Here's how the part is built. I have some questions about the finished solid (model axes, mm). Face numbers are marked on the shaded views. A direction names the side the tool comes from. Give positions to 0.01 mm unless a question says otherwise; leave off trailing zeros. Write each loop counter-clockwise with the first axis right and the second up, starting at its lowest first coordinate (ties: lowest second). Pieces come first, ordered by that corner, then holes. Notation, with made-up numbers: (76, 53.5) - (94, 53.5) arc R24 ccw to (94, 83.5) - close; hole circle Ø11 at (-18.5, 45). An arc over 180 degrees is marked (long way). One line per item, written item: value. Start each with the question number.
1) Imagine slicing it at A-A on x = 62.5. Write out the boundary of the cut face in (y, z).
2) Imagine slicing it at C-C on y = -21. Write out the boundary of the cut face in (x, z), plus the area to 3 significant figures.
3) On a 3-axis mill with a long thin cutter (end or side, diameter ignored), from which of +Z, -Z, +X, -X, +Y, -Y can I reach the whole of each face in a straight line? I mean the marked faces 4 and 5. Say none if no direction works.
4) Please list where these lines run through material, in increasing order: L1, parallel to Y at x = -0.95, z = 0; L2, parallel to Y at x = 6, z = 0; L3, parallel to Z at x = 6, y = -21. Write a range as [from, to].
5) Imagine slicing it at B-B on y = 42. Write out the boundary of the cut face in (x, z).
6) We'd pull the mould along Y, two halves only. Please class the marked faces 1, 2 and 3: +Y half, -Y half, draft (parallel to the pull), parting line (faces both ways), or undercut.
7) Imagine slicing it at D-D on z = -27. Write out the boundary of the cut face in (x, y), plus the area to 3 significant figures.
8) I'm going to push flat-ended pins straight in: P1, Ø1.4, axis at x = 64, y = 7, coming from the -Z side; P2, Ø13.5, axis at y = -3.5, z = -0.5, coming from the -X side; P3, Ø1.3, axis at x = 66.5, z = -1, coming from the +Y side; P4, Ø4.5, axis at y = 29, z = 0, coming from the -X side. Where does each tip first touch, or does it pass through?
from build123d import *

# Parameters (mm, degrees)
ESQUISSE3_R             = 3
ENL_V_MAT_EXTRU_1_DEPTH = 102.901913623
ESQUISSE7_R             = 3
ENL_V_MAT_EXTRU_2_DEPTH = 102.901913623
TROU_TARAUD_M63_D       = 5
TROU_TARAUD_M63_DEPTH   = 15
TROU_TARAUD_M63_TIP     = 1.502151548
D_GAGEMENT_M37_REACH    = 105.064
D_GAGEMENT_M37_BORE_R   = 1.7
ESQUISSE6_W             = 10.447703872
ESQUISSE6_H             = 4.5
ENL_V_MAT_EXTRU_3_DEPTH = 2
D_GAGEMENT_M51_D        = 5.5
D_GAGEMENT_M51_DEPTH    = 12
D_GAGEMENT_M51_TIP      = 1.652366702


with BuildPart() as part:
    # Esquisse1 → Révolution2 (revolve)
    with BuildSketch(Plane.XY, mode=Mode.PRIVATE) as r_volution2_sk:
        with BuildLine():
            Line((0, 0), (74.5, 0))
            Line((74.5, 0), (74.5, -6))
            Line((74.5, -6), (69.5, -6))
            Line((69.5, -6), (69.5, -7))
            Line((69.5, -7), (68, -8.5))
            Line((68, -8.5), (60.5, -8.5))
            Line((60.5, -8.5), (60.5, -7.5))
            Line((60.5, -7.5), (59.5, -7.5))
            Line((59.5, -7.5), (59.5, -10))
            Line((59.5, -10), (13, -10))
            ThreePointArc((13, -10), (12.646446609, -10.146446609), (12.5, -10.5))
            Line((12.5, -10.5), (12.5, -13.5))
            Line((12.5, -13.5), (8.5, -17))
            Line((8.5, -17), (8.5, -48))
            Line((8.5, -48), (-1.5, -48))
            Line((-1.5, -48), (-1.5, -35))
            Line((-1.5, -35), (0, -35))
            Line((0, -35), (0, 0))
        make_face()
    revolve(r_volution2_sk.sketch.rotate(Axis((-50.843487897, 0, 0), (1, 0, 0)), 270), axis=Axis((-50.843487897, 0, 0), (1, 0, 0)))

    # Esquisse2 → Dégagement M32 (revolve, cut)
    with BuildSketch(Plane(origin=(74.5, 0, 0), x_dir=(0, 0, -1), z_dir=(0, 1, 0))):
        Polygon((0, 0), (0, 14.981495458), (1.7, 14), (1.7, 0), align=None)
    revolve(axis=Axis((80.85, 0, 0), (-1, 0, 0)), mode=Mode.SUBTRACT)

    # Esquisse3 → Enlèv. mat.-Extru.1 (cut, through all)
    with BuildSketch(Plane.ZY.offset(1.5)):
        with Locations((-40, 0)):
            Circle(ESQUISSE3_R)
        with Locations((40, 0)):
            Circle(ESQUISSE3_R)
    extrude(amount=-ENL_V_MAT_EXTRU_1_DEPTH, mode=Mode.SUBTRACT)

    # Esquisse7 → Enlèv. mat.-Extru.2 (cut, through all)
    with BuildSketch(Plane.ZY.offset(1.5)):
        with Locations((0, -44)):
            Circle(ESQUISSE7_R)
    extrude(amount=-ENL_V_MAT_EXTRU_2_DEPTH, mode=Mode.SUBTRACT)

    # Trou taraudé M63
    with Locations(Plane(origin=(-1.5, 42, 0), x_dir=(0, 0, -1), z_dir=(-1, 0, 0))):
        with Locations((0, 0), (36.373066959, 63), (-36.373066959, 63)):
            Hole(TROU_TARAUD_M63_D / 2, depth=TROU_TARAUD_M63_DEPTH)
            with Locations((0, 0, -(TROU_TARAUD_M63_DEPTH + TROU_TARAUD_M63_TIP / 2))):  # 118° drill point
                Cone(0, TROU_TARAUD_M63_D / 2, TROU_TARAUD_M63_TIP, mode=Mode.SUBTRACT)

    # Dégagement M37 bore (on position points) → Dégagement M37 (cut, up to next)
    with BuildSketch(Plane(origin=(72, 6, 0), x_dir=(0, 0, 1), z_dir=(0, 1, 0)), mode=Mode.PRIVATE) as d_gagement_m37_sk1:
        Circle(D_GAGEMENT_M37_BORE_R)
    d_gagement_m37_tool1 = extrude(d_gagement_m37_sk1.sketch, amount=-D_GAGEMENT_M37_REACH, mode=Mode.PRIVATE) & part.part
    add(d_gagement_m37_tool1.solids().sort_by_distance((72, 6, 0))[0], mode=Mode.SUBTRACT)

    # Esquisse6 → Enlèv. mat.-Extru.3 (cut)
    with BuildSketch(Plane(origin=(0, 8.5, 0), x_dir=(-1, 0, 0), z_dir=(0, 1, 0))):
        with Locations((-65.723851936, 0)):
            Rectangle(ESQUISSE6_W, ESQUISSE6_H)
    extrude(amount=-ENL_V_MAT_EXTRU_3_DEPTH, mode=Mode.SUBTRACT)

    # Dégagement M51
    with Locations(Plane(origin=(8.5, 29, 0), x_dir=(0, 0, 1), z_dir=(1, 0, 0))):
        with Locations((0, 0)):
            Hole(D_GAGEMENT_M51_D / 2, depth=D_GAGEMENT_M51_DEPTH)
            with Locations((0, 0, -(D_GAGEMENT_M51_DEPTH + D_GAGEMENT_M51_TIP / 2))):  # 118° drill point
                Cone(0, D_GAGEMENT_M51_D / 2, D_GAGEMENT_M51_TIP, mode=Mode.SUBTRACT)


solid = part.part
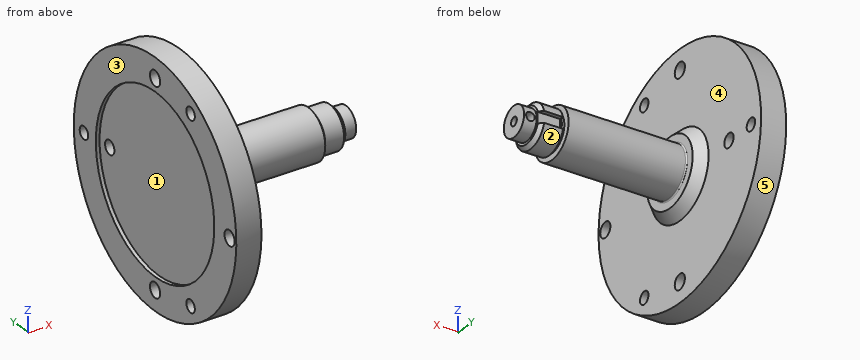
Numbers:
1. outline: (6.5, -2.25) - (6.5, 2.25) - (8.2, 2.25) arc R8.5 ccw (long way) to (8.2, -2.25) - close; hole circle Ø3.4 at (0, 0)
2. outline: (-1.5, -43.16) - (8.5, -43.16) - (8.5, -38.87) - (-1.5, -38.87) - close; (-1.5, -33.87) - (8.5, -33.87) - (8.5, 33.87) - (-1.5, 33.87) - (-1.5, 28) - (0, 28) - (0, -28) - (-1.5, -28) - close; (-1.5, 38.87) - (8.5, 38.87) - (8.5, 43.16) - (-1.5, 43.16) - close
2. area: 679 mm^2
3. face 4: +X
3. face 5: +X, -X
4. L1: [-48, -47], [-41, -35], [35, 39.5], [44.5, 48]
4. L2: [-48, -47], [-41, 26.25], [31.75, 39.5], [44.5, 48]
4. L3: [-43.16, -38.87], [-33.87, 33.87], [38.87, 43.16]
5. outline: (-1.5, -23.24) - (8.5, -23.24) - (8.5, -2.5) - (-1.5, -2.5) - close; (-1.5, 2.5) - (8.5, 2.5) - (8.5, 23.24) - (-1.5, 23.24) - close
6. face 1: undercut
6. face 2: parting line
6. face 3: draft
7. outline: (-1.5, -39.69) - (8.5, -39.69) - (8.5, 39.69) - (-1.5, 39.69) - (-1.5, 22.27) - (0, 22.27) - (0, -22.27) - (-1.5, -22.27) - close
7. area: 727 mm^2
8. P1: z = -5.71
8. P2: x = 0
8. P3: y = 6.5
8. P4: through
